Could you check a few things on this drawing? It's one solid part, dimensions in mm from its lowest x, y, z. Give positions to 0.01 mm unless a question says otherwise; leave off trailing zeros. Order: outer loops, then holes, each group sorted by start corner. A loop starts at its lowest first (then second) coordinate and runs counter-clockwise, first axis right, second up.
(1) Imagine slicing it at A-A, the plane x = 4.5. Write out the boundary of the cut face in (y, z), then the cut area to 3 significant figures.
(2) Imagine slicing it at C-C, the plane y = 2. Write out the boundary of the cut face in (x, z), then the cut area to 3 significant figures.
(3) If I drill on probe 1 along Y at (x, z) = (4.5, 1.9); probe 2 along Y at (x, z) = (7, 1), over which ranges is the centre line in solid material (lowest first)?
(4) Imagine slicing it at B-B, the plane z = 2.65. State how many separate pieces and enclosed holes the cut face has, then the cut area to 3 significant figures.
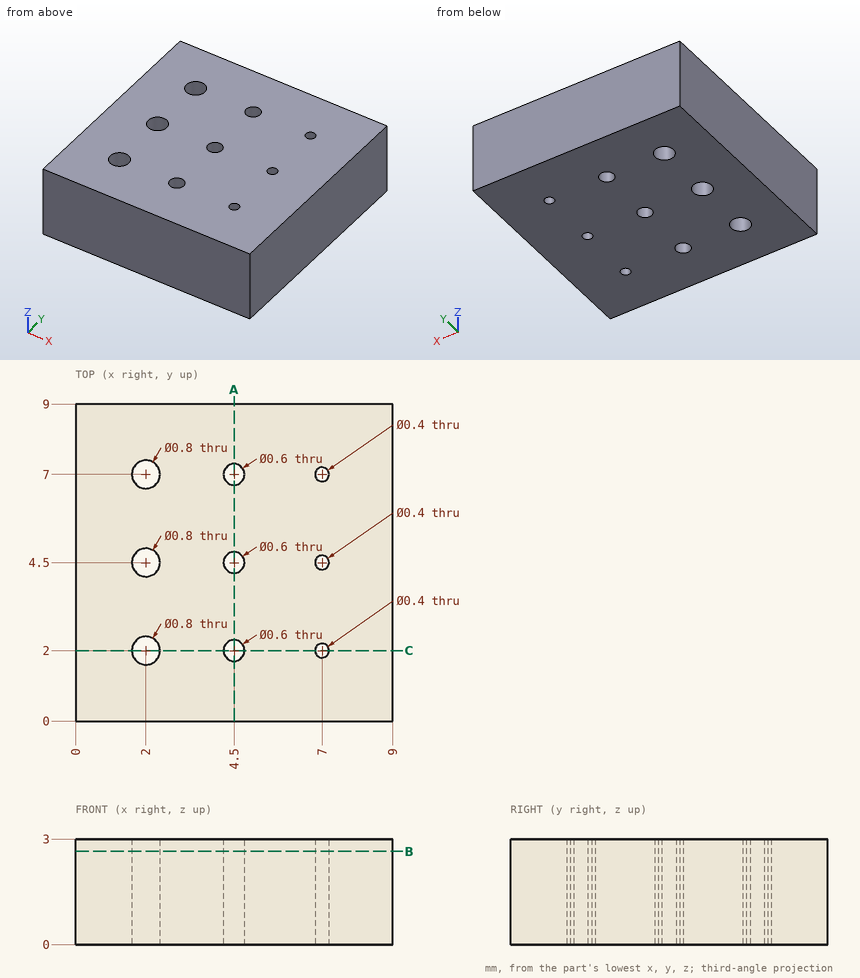
Answer block:
1. outline: (0, 0) - (1.7, 0) - (1.7, 3) - (0, 3) - close; (2.3, 0) - (4.2, 0) - (4.2, 3) - (2.3, 3) - close; (4.8, 0) - (6.7, 0) - (6.7, 3) - (4.8, 3) - close; (7.3, 0) - (9, 0) - (9, 3) - (7.3, 3) - close
1. area: 21.6 mm2
2. outline: (0, 0) - (1.6, 0) - (1.6, 3) - (0, 3) - close; (2.4, 0) - (4.2, 0) - (4.2, 3) - (2.4, 3) - close; (4.8, 0) - (6.8, 0) - (6.8, 3) - (4.8, 3) - close; (7.2, 0) - (9, 0) - (9, 3) - (7.2, 3) - close
2. area: 21.6 mm2
3. probe 1: y = 0 to 1.7, 2.3 to 4.2, 4.8 to 6.7, 7.3 to 9
3. probe 2: y = 0 to 1.8, 2.2 to 4.3, 4.7 to 6.8, 7.2 to 9
4. separate pieces: 1
4. enclosed holes: 9
4. area: 78.3 mm2
